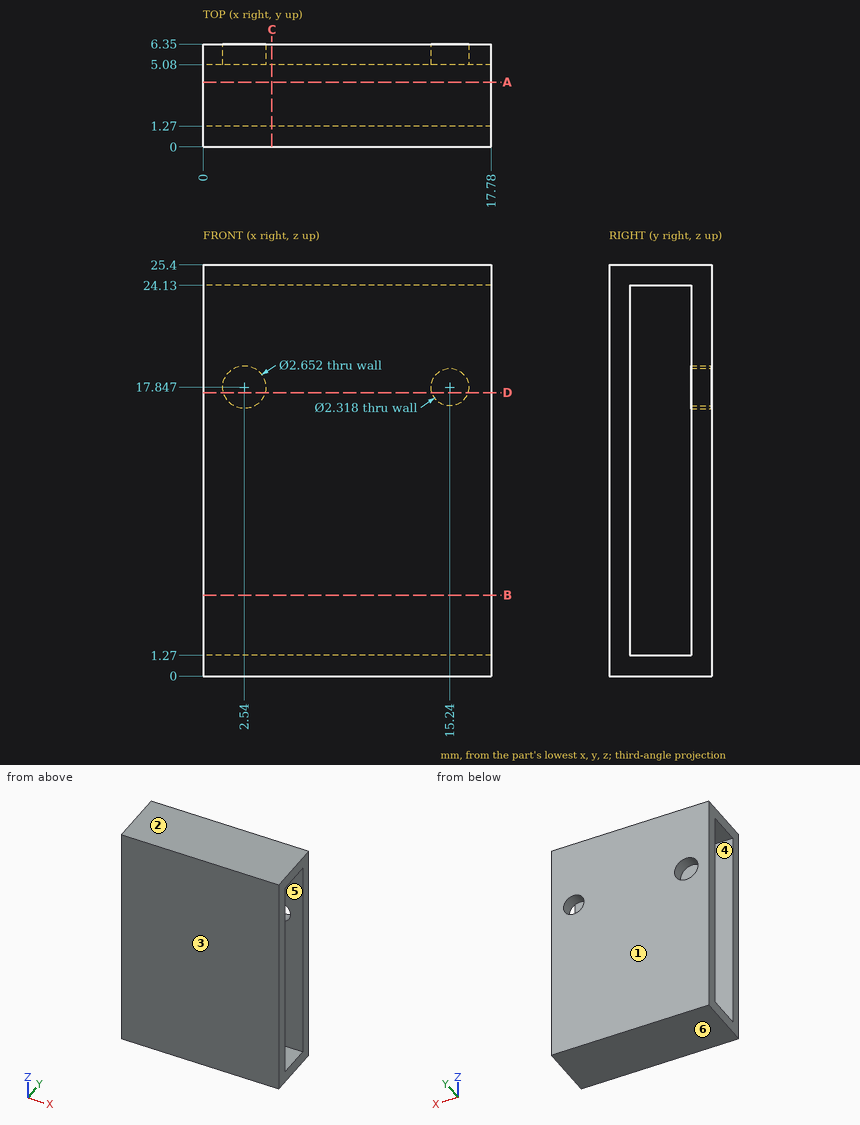
Check sheet for the drawn part. Datum: minimum x, y, z corner. Units: mm. A direction names the side the tool comes from. Round coordinates to 2 decimals unless told otherwise and drop trailing zeros. Order: outer loops, then holes, each group sorted by start corner. A loop starts at its lowest first (then second) coordinate and runs counter-clockwise, first axis right, second up.
1) Section check C-C (x = 4.25). Record the boundary of the cut face in (y, z).
2) Section check B-B (z = 5). Record the boundary of the cut face in (x, y).
3) Tool access check on the marked faces 5 and 6. Record the directions out of +Z, -Z, +X, -X, +Y, -Y that give a thin tool (end or side, any length) a straight path to the whole face; none if there is none.
4) Mould release check, pull along Y, two halves, no side actions. Record for the marked faces 1, 2, 3 and 4: +Y half, -Y half, draft (parallel to the pull), parting line (faces both ways), or undercut.
5) Scan lines: line 1 (Y direction, x = 13, z = 9); line 2 (Z direction, x = 15.24, y = 5.95); line 3 (Z direction, x = 2.54, y = 6.15). Record each from-to range of solid material in increasing order.
6) Section check A-A (y = 4). Record the boundary of the cut face in (x, z).
7) Section check D-D (z = 17.5). Record the boundary of the cut face in (x, y).
Result:
1. outline: (0, 0) - (6.35, 0) - (6.35, 25.4) - (0, 25.4) - close; hole (1.27, 1.27) - (5.08, 1.27) - (5.08, 24.13) - (1.27, 24.13) - close
2. outline: (0, 0) - (17.78, 0) - (17.78, 1.27) - (0, 1.27) - close; (0, 5.08) - (17.78, 5.08) - (17.78, 6.35) - (0, 6.35) - close
3. face 5: +X, -X
3. face 6: -Z, +X, -X, +Y, -Y
4. face 1: +Y half
4. face 2: draft
4. face 3: -Y half
4. face 4: undercut
5. line 1: y = 0 to 1.27, 5.08 to 6.35
5. line 2: z = 0 to 16.69, 19.01 to 25.4
5. line 3: z = 0 to 16.52, 19.17 to 25.4
6. outline: (0, 0) - (17.78, 0) - (17.78, 1.27) - (0, 1.27) - close; (0, 24.13) - (17.78, 24.13) - (17.78, 25.4) - (0, 25.4) - close
7. outline: (0, 0) - (17.78, 0) - (17.78, 1.27) - (0, 1.27) - close; (0, 5.08) - (1.26, 5.08) - (1.26, 6.35) - (0, 6.35) - close; (3.82, 5.08) - (14.13, 5.08) - (14.13, 6.35) - (3.82, 6.35) - close; (16.35, 5.08) - (17.78, 5.08) - (17.78, 6.35) - (16.35, 6.35) - close
